Here's the drawing with two shaded views (mm, measured from the low corner). I have some questions. Round coordinates to 2 decimals unless told otherwise and drop trailing zeros. Loops run counter-clockwise (first coordinate to the right, second up) from the corner with the lowest first, then second, coordinate; pieces in that order, holes last.
(1) I want a section at D-D on z = 0.75. Write out the boundary of the cut face in (x, y).
(2) Will these pins go through, and if not, where does the flat tip stop? pin 1 Ø2.5 at (x, y) = (23, 8.5) entering from -Z; pin 2 Ø5 at (x, y) = (33, 8.5) entering from +Z; pin 3 Ø0.8 at (y, z) = (32.5, 1) entering from +X.
(3) If I drill on line 1 along Y through (x, z) = (8, 0.55); line 2 along Y through (x, z) = (25, 0.4); line 3 along X through (y, z) = (7.5, 0.45), over which ranges is the centre line in solid material (lowest first)?
(4) I want a section at A-A on x = 23. Write out the boundary of the cut face in (y, z), plus the area to 3 significant figures.
(5) I want a section at B-B on x = 19. Write out the boundary of the cut face in (y, z), plus the area to 3 significant figures.
(6) I want a section at C-C on y = 8.5. Write out the boundary of the cut face in (x, z), plus the area to 3 significant figures.
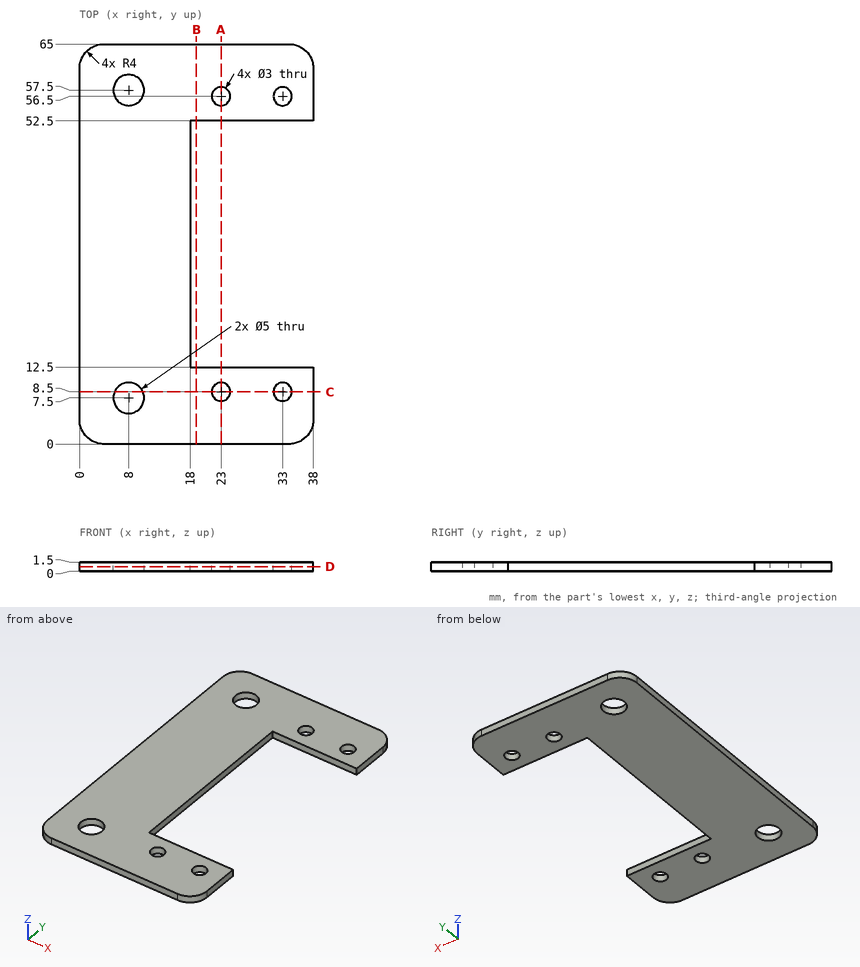
Filled sheet:
1. outline: (0, 4) arc R4 ccw to (4, 0) - (34, 0) arc R4 ccw to (38, 4) - (38, 12.5) - (18, 12.5) - (18, 52.5) - (38, 52.5) - (38, 61) arc R4 ccw to (34, 65) - (4, 65) arc R4 ccw to (0, 61) - close; hole circle Ø5 at (8, 7.5); hole circle Ø5 at (8, 57.5); hole circle Ø3 at (23, 8.5); hole circle Ø3 at (23, 56.5); hole circle Ø3 at (33, 8.5); hole circle Ø3 at (33, 56.5)
2. pin 1: passes through
2. pin 2: stops at z = 1.5
2. pin 3: stops at x = 18
3. line 1: y = 0 to 5, 10 to 55, 60 to 65
3. line 2: y = 0 to 12.5, 52.5 to 65
3. line 3: x = 0 to 5.5, 10.5 to 21.88, 24.12 to 31.88, 34.12 to 38
4. outline: (0, 0) - (7, 0) - (7, 1.5) - (0, 1.5) - close; (10, 0) - (12.5, 0) - (12.5, 1.5) - (10, 1.5) - close; (52.5, 0) - (55, 0) - (55, 1.5) - (52.5, 1.5) - close; (58, 0) - (65, 0) - (65, 1.5) - (58, 1.5) - close
4. area: 28.5 mm2
5. outline: (0, 0) - (12.5, 0) - (12.5, 1.5) - (0, 1.5) - close; (52.5, 0) - (65, 0) - (65, 1.5) - (52.5, 1.5) - close
5. area: 37.5 mm2
6. outline: (0, 0) - (5.71, 0) - (5.71, 1.5) - (0, 1.5) - close; (10.29, 0) - (21.5, 0) - (21.5, 1.5) - (10.29, 1.5) - close; (24.5, 0) - (31.5, 0) - (31.5, 1.5) - (24.5, 1.5) - close; (34.5, 0) - (38, 0) - (38, 1.5) - (34.5, 1.5) - close
6. area: 41.1 mm2
